```python
from build123d import *

# Parameters (mm, degrees)
CUT_EXTRUDE1_REACH = 29.699
CUT_EXTRUDE2_REACH = 29.699


with BuildPart() as part:
    # Sketch1 → Revolve1 (revolve)
    with BuildSketch(Plane.XY, mode=Mode.PRIVATE) as revolve1_sk:
        Polygon((12.7, 17.399), (13.462, 14.859), (12.7, 14.859), (12.7, 11.43), (15.24, 11.43), (15.24, 8.89), (9.779, 8.89), (9.779, 2.54), (10.541, 2.54), (9.779, 0), (7.239, 0), (7.239, 11.43), (10.16, 11.43), (10.16, 17.399), align=None)
    revolve(revolve1_sk.sketch.rotate(Axis((0, 0, 0), (0, 1, 0)), 90), axis=Axis((0, 0, 0), (0, 1, 0)))

    # Cut-Extrude1: up to this face of the body (flat: up to its plane)
    cut_extrude1_end = Plane(part.part.faces().sort_by_distance((0, 11.43, 13.131052294))[0])
    # Sketch2 → Cut-Extrude1 (cut, up to the picked face)
    with BuildSketch(Plane(origin=(0, 17.399, 0), x_dir=(1, 0, 0), z_dir=(0, 1, 0)), mode=Mode.PRIVATE) as cut_extrude1_sk1:
        with BuildLine():
            Line((-9.418572079, 3.81), (-12.911597268, 3.81))
            ThreePointArc((-12.911597268, 3.81), (-9.519071488, 9.519071488), (-3.81, 12.911597268))
            Line((-3.81, 12.911597268), (-3.81, 9.418572079))
            ThreePointArc((-3.81, 9.418572079), (-7.184204897, 7.184204897), (-9.418572079, 3.81))
        make_face()
    cut_extrude1_tool1 = split(extrude(cut_extrude1_sk1.sketch, amount=-CUT_EXTRUDE1_REACH, mode=Mode.PRIVATE), bisect_by=cut_extrude1_end, keep=Keep.BOTH, mode=Mode.PRIVATE)
    # Sketch2 → Cut-Extrude1 (cut, up to the picked face)
    with BuildSketch(Plane(origin=(0, 17.399, 0), x_dir=(1, 0, 0), z_dir=(0, 1, 0)), mode=Mode.PRIVATE) as cut_extrude1_sk2:
        with BuildLine():
            Line((-12.911597268, -3.81), (-9.418572079, -3.81))
            ThreePointArc((-9.418572079, -3.81), (-7.184204897, -7.184204897), (-3.81, -9.418572079))
            Line((-3.81, -9.418572079), (-3.81, -12.911597268))
            ThreePointArc((-3.81, -12.911597268), (-9.519071488, -9.519071488), (-12.911597268, -3.81))
        make_face()
    cut_extrude1_tool2 = split(extrude(cut_extrude1_sk2.sketch, amount=-CUT_EXTRUDE1_REACH, mode=Mode.PRIVATE), bisect_by=cut_extrude1_end, keep=Keep.BOTH, mode=Mode.PRIVATE)
    # Sketch2 → Cut-Extrude1 (cut, up to the picked face)
    with BuildSketch(Plane(origin=(0, 17.399, 0), x_dir=(1, 0, 0), z_dir=(0, 1, 0)), mode=Mode.PRIVATE) as cut_extrude1_sk3:
        with BuildLine():
            Line((3.81, 9.418572079), (3.81, 12.911597268))
            ThreePointArc((3.81, 12.911597268), (9.519071488, 9.519071488), (12.911597268, 3.81))
            Line((12.911597268, 3.81), (9.418572079, 3.81))
            ThreePointArc((9.418572079, 3.81), (7.184204897, 7.184204897), (3.81, 9.418572079))
        make_face()
    cut_extrude1_tool3 = split(extrude(cut_extrude1_sk3.sketch, amount=-CUT_EXTRUDE1_REACH, mode=Mode.PRIVATE), bisect_by=cut_extrude1_end, keep=Keep.BOTH, mode=Mode.PRIVATE)
    # Sketch2 → Cut-Extrude1 (cut, up to the picked face)
    with BuildSketch(Plane(origin=(0, 17.399, 0), x_dir=(1, 0, 0), z_dir=(0, 1, 0)), mode=Mode.PRIVATE) as cut_extrude1_sk4:
        with BuildLine():
            Line((9.418572079, -3.81), (12.911597268, -3.81))
            ThreePointArc((12.911597268, -3.81), (9.519071488, -9.519071488), (3.81, -12.911597268))
            Line((3.81, -12.911597268), (3.81, -9.418572079))
            ThreePointArc((3.81, -9.418572079), (7.184204897, -7.184204897), (9.418572079, -3.81))
        make_face()
    cut_extrude1_tool4 = split(extrude(cut_extrude1_sk4.sketch, amount=-CUT_EXTRUDE1_REACH, mode=Mode.PRIVATE), bisect_by=cut_extrude1_end, keep=Keep.BOTH, mode=Mode.PRIVATE)
    add(cut_extrude1_tool1.solids().sort_by(Axis((-8.150135, 17.399, -8.150135), (0, -1, 0)))[0], mode=Mode.SUBTRACT)
    add(cut_extrude1_tool2.solids().sort_by(Axis((-8.150135, 17.399, 8.150135), (0, -1, 0)))[0], mode=Mode.SUBTRACT)
    add(cut_extrude1_tool3.solids().sort_by(Axis((8.150135, 17.399, -8.150135), (0, -1, 0)))[0], mode=Mode.SUBTRACT)
    add(cut_extrude1_tool4.solids().sort_by(Axis((8.150135, 17.399, 8.150135), (0, -1, 0)))[0], mode=Mode.SUBTRACT)

    # Cut-Extrude2: up to this face of the body (flat: up to its plane)
    cut_extrude2_end = Plane(part.part.faces().sort_by_distance((0, 8.89, 14.808947706))[0])
    # Sketch3 → Cut-Extrude2 (cut, up to the picked face)
    with BuildSketch(Plane.XZ, mode=Mode.PRIVATE) as cut_extrude2_sk1:
        with BuildLine():
            Line((-6.505574225, 3.175), (-10.05147034, 3.175))
            ThreePointArc((-10.05147034, 3.175), (-7.45361258, 7.45361258), (-3.175, 10.05147034))
            Line((-3.175, 10.05147034), (-3.175, 6.505574225))
            ThreePointArc((-3.175, 6.505574225), (-5.118745989, 5.118745989), (-6.505574225, 3.175))
        make_face()
    cut_extrude2_tool1 = split(extrude(cut_extrude2_sk1.sketch, amount=-CUT_EXTRUDE2_REACH, mode=Mode.PRIVATE), bisect_by=cut_extrude2_end, keep=Keep.BOTH, mode=Mode.PRIVATE)
    # Sketch3 → Cut-Extrude2 (cut, up to the picked face)
    with BuildSketch(Plane.XZ, mode=Mode.PRIVATE) as cut_extrude2_sk2:
        with BuildLine():
            Line((-6.505574225, -3.175), (-10.05147034, -3.175))
            ThreePointArc((-10.05147034, -3.175), (-7.45361258, -7.45361258), (-3.175, -10.05147034))
            Line((-3.175, -10.05147034), (-3.175, -6.505574225))
            ThreePointArc((-3.175, -6.505574225), (-5.118745989, -5.118745989), (-6.505574225, -3.175))
        make_face()
    cut_extrude2_tool2 = split(extrude(cut_extrude2_sk2.sketch, amount=-CUT_EXTRUDE2_REACH, mode=Mode.PRIVATE), bisect_by=cut_extrude2_end, keep=Keep.BOTH, mode=Mode.PRIVATE)
    # Sketch3 → Cut-Extrude2 (cut, up to the picked face)
    with BuildSketch(Plane.XZ, mode=Mode.PRIVATE) as cut_extrude2_sk3:
        with BuildLine():
            Line((3.175, 6.505574225), (3.175, 10.05147034))
            ThreePointArc((3.175, 10.05147034), (7.45361258, 7.45361258), (10.05147034, 3.175))
            Line((10.05147034, 3.175), (6.505574225, 3.175))
            ThreePointArc((6.505574225, 3.175), (5.118745989, 5.118745989), (3.175, 6.505574225))
        make_face()
    cut_extrude2_tool3 = split(extrude(cut_extrude2_sk3.sketch, amount=-CUT_EXTRUDE2_REACH, mode=Mode.PRIVATE), bisect_by=cut_extrude2_end, keep=Keep.BOTH, mode=Mode.PRIVATE)
    # Sketch3 → Cut-Extrude2 (cut, up to the picked face)
    with BuildSketch(Plane.XZ, mode=Mode.PRIVATE) as cut_extrude2_sk4:
        with BuildLine():
            Line((6.505574225, -3.175), (10.05147034, -3.175))
            ThreePointArc((10.05147034, -3.175), (7.45361258, -7.45361258), (3.175, -10.05147034))
            Line((3.175, -10.05147034), (3.175, -6.505574225))
            ThreePointArc((3.175, -6.505574225), (5.118745989, -5.118745989), (6.505574225, -3.175))
        make_face()
    cut_extrude2_tool4 = split(extrude(cut_extrude2_sk4.sketch, amount=-CUT_EXTRUDE2_REACH, mode=Mode.PRIVATE), bisect_by=cut_extrude2_end, keep=Keep.BOTH, mode=Mode.PRIVATE)
    add(cut_extrude2_tool1.solids().sort_by(Axis((-6.228446, 0, 6.228446), (0, 1, 0)))[0], mode=Mode.SUBTRACT)
    add(cut_extrude2_tool2.solids().sort_by(Axis((-6.228446, 0, -6.228446), (0, 1, 0)))[0], mode=Mode.SUBTRACT)
    add(cut_extrude2_tool3.solids().sort_by(Axis((6.228446, 0, 6.228446), (0, 1, 0)))[0], mode=Mode.SUBTRACT)
    add(cut_extrude2_tool4.solids().sort_by(Axis((6.228446, 0, -6.228446), (0, 1, 0)))[0], mode=Mode.SUBTRACT)


solid = part.part
```
The model under review builds one solid part; all positions refer to its coordinate system, in mm. A direction names the side the tool comes from. Round coordinates to 2 decimals unless told otherwise and drop trailing zeros. Order: outer loops, then holes, each group sorted by start corner. A loop starts at its lowest first (then second) coordinate and runs counter-clockwise, first axis right, second up. Notation, with made-up numbers: (-5, 21) -> (49, 21) arc R21 cw to (49, 50) -> close; hole circle Ø11 at (2, 66). An arc over 180 degrees is marked (long way). One line per item, written item: value. Start each with the question number.
Q1. Take a section at C-C (y = 14.25). Write out the cut boundary in (x, z).
Q2. Take a section at B-B (x = 0). Write out the cut boundary in (y, z), and give its area (3 significant figures).
Q3. Take a section at A-A (z = 0). Write out the cut boundary in (x, y), and give its area (3 significant figures).
Q4. Take a section at D-D (y = 8.25). Write out the cut boundary in (x, z) (3 decimals), and give its area (3 significant figures).
Q5. Wall thickness on line 1 (X direction, y = 4, z = 0); line 2 (X direction, y = 15.5, z = 11); line 3 (Z direction, x = 1, y = 7.5): over which ranges is each line inside the solid? List them lowest first.
Q6. Machinability: for faces 1 (the face through (3.175, 4, -8)), 2 (the face through (-11, 14, 3.81)), 3 (the face through (10.16, 14.46, 0.05)), 4 (the face through (-8, 4, 3.175)), which of the approach directions +Z, -Z, +X, -X, +Y, -Y give a long, thin tool a straight path to every point of the face, cutting with its end or side? Answer none if there is none.
Q7. Mouldability with a two-part tool opening along Y and no side actions: class faces 5 (the face through (10.155, 1.252, 0.047)), 6 (the face through (3.81, 14, 11)), 7 (the face through (0.05, 5.67, -9.78)), 8 (the face through (-11, 17.399, 0)) as released by +Y, released by -Y, zero draft, split by the parting line, or undercut.
Q8. Clearance check with flat-ended pins moving along their axes: pin 1 Ø4 at (x, y) = (7.5, 3.5) entering from +Z (3 decimals); pin 2 Ø1.7 at (x, y) = (11, 14.5) entering from +Z; pin 3 Ø3 at (y, z) = (4.5, -8.5) entering from -X (3 decimals). State where each tip first meets the part, or that it passes through.
Reported:
1. outline: (-12.12, -3.81) -> (-9.42, -3.81) arc R10.16 cw to (-9.42, 3.81) -> (-12.12, 3.81) arc R12.7 ccw to start; (-3.81, -12.12) arc R12.7 ccw to (3.81, -12.12) -> (3.81, -9.42) arc R10.16 cw to (-3.81, -9.42) -> close; (-3.81, 9.42) arc R10.16 cw to (3.81, 9.42) -> (3.81, 12.12) arc R12.7 ccw to (-3.81, 12.12) -> close; (9.42, -3.81) -> (12.12, -3.81) arc R12.7 ccw to (12.12, 3.81) -> (9.42, 3.81) arc R10.16 cw to start
2. outline: (0, -9.78) -> (2.54, -10.54) -> (2.54, -9.78) -> (8.89, -9.78) -> (8.89, -15.24) -> (11.43, -15.24) -> (11.43, -12.7) -> (14.86, -12.7) -> (14.86, -13.46) -> (17.4, -12.7) -> (17.4, -10.16) -> (11.43, -10.16) -> (11.43, -7.24) -> (0, -7.24) -> close; (0, 7.24) -> (11.43, 7.24) -> (11.43, 10.16) -> (17.4, 10.16) -> (17.4, 12.7) -> (14.86, 13.46) -> (14.86, 12.7) -> (11.43, 12.7) -> (11.43, 15.24) -> (8.89, 15.24) -> (8.89, 9.78) -> (2.54, 9.78) -> (2.54, 10.54) -> (0, 9.78) -> close
2. area: 120 mm2
3. outline: (-15.24, 8.89) -> (-9.78, 8.89) -> (-9.78, 2.54) -> (-10.54, 2.54) -> (-9.78, 0) -> (-7.24, 0) -> (-7.24, 11.43) -> (-10.16, 11.43) -> (-10.16, 17.4) -> (-12.7, 17.4) -> (-13.46, 14.86) -> (-12.7, 14.86) -> (-12.7, 11.43) -> (-15.24, 11.43) -> close; (7.24, 0) -> (9.78, 0) -> (10.54, 2.54) -> (9.78, 2.54) -> (9.78, 8.89) -> (15.24, 8.89) -> (15.24, 11.43) -> (12.7, 11.43) -> (12.7, 14.86) -> (13.46, 14.86) -> (12.7, 17.4) -> (10.16, 17.4) -> (10.16, 11.43) -> (7.24, 11.43) -> close
3. area: 120 mm2
4. outline: (-9.249, -3.175) -> (-6.506, -3.175) arc R7.239 cw to (-6.506, 3.175) -> (-9.249, 3.175) arc R9.779 ccw to start; (-3.175, -9.249) arc R9.779 ccw to (3.175, -9.249) -> (3.175, -6.506) arc R7.239 cw to (-3.175, -6.506) -> close; (-3.175, 6.506) arc R7.239 cw to (3.175, 6.506) -> (3.175, 9.249) arc R9.779 ccw to (-3.175, 9.249) -> close; (6.506, -3.175) -> (9.249, -3.175) arc R9.779 ccw to (9.249, 3.175) -> (6.506, 3.175) arc R7.239 cw to start
4. area: 66.2 mm2
5. line 1: x = -9.78 to -7.24, 7.24 to 9.78
5. line 2: x = -3.81 to 3.81
5. line 3: z = -9.73 to -7.17, 7.17 to 9.73
6. face 1: +Z, -Z, +X, -Y
6. face 2: +Z, +X, -X, +Y
6. face 3: +Y
6. face 4: +Z, +X, -X, -Y
7. face 5: released by -Y
7. face 6: zero draft
7. face 7: undercut
7. face 8: released by +Y
8. pin 1: stops at z = 3.175
8. pin 2: stops at z = 3.81
8. pin 3: stops at x = -3.175
